Geometry check sheet. Reference: the model listing, model coordinates, mm. Face numbers are marked on the shaded views. A direction names the side the tool comes from. Round coordinates to 2 decimals unless told otherwise and drop trailing zeros. Loops run counter-clockwise (first coordinate to the right, second up) from the corner with the lowest first, then second, coordinate; pieces in that order, holes last.
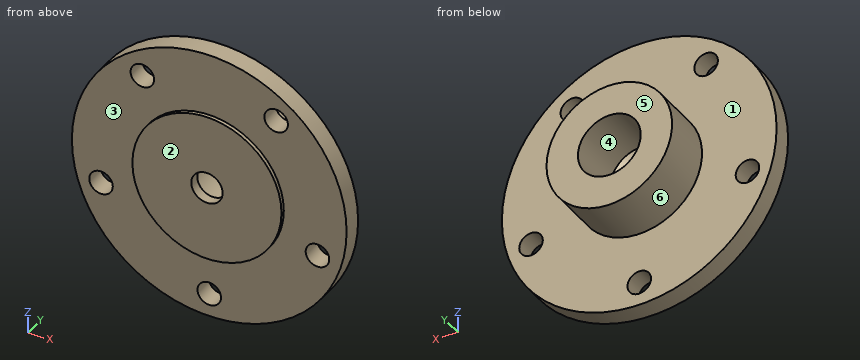
Autodesk Inventor part; units mm, degrees
ref_plane "YZ Plane" through (0, 0, 0) normal (1, 0, 0) x (0, 1, 0)
ref_plane "XZ Plane" through (0, 0, 0) normal (0, 1, 0) x (-1, 0, 0)
ref_plane "XY Plane" through (0, 0, 0) normal (0, 0, 1) x (1, 0, 0)
sketch "Sketch1" plane through (0, 0, 0) normal (0, 1, 0) x (-1, 0, 0)
  circle A0 centre (0, 0) radius 17.5
  dimension "d0" = 35
extrude "Extrusion1" add sketch "Sketch1" along normal mid plane 2.5
sketch "Sketch2" plane through (0, 1.25, 0) normal (0, 1, 0) x (1, 0, 0)
  circle A0 centre (0, 0) radius 8
  dimension "d3" = 16
extrude "Extrusion2" add sketch "Sketch2" along normal blind 6.5
sketch "Sketch3" plane through (0, -1.25, 0) normal (0, -1, 0) x (1, 0, 0)
  circle A0 centre (0, 0) radius 9.5
  dimension "d6" = 19
extrude "Extrusion3" add sketch "Sketch3" along normal blind 0.5
sketch "Sketch6" plane through (0, 1.25, 0) normal (0, 1, 0) x (1, 0, 0)
  circle A0 centre (0, 14.5) radius 1.5
  circle A1 centre (-13.7903, 4.4807) radius 1.5
  circle A2 centre (-8.5229, -11.7307) radius 1.5
  circle A3 centre (8.5229, -11.7307) radius 1.5
  circle A4 centre (13.7903, 4.4807) radius 1.5
  point P0 (0, 0)
  dimension "d17" = 3
  dimension "d18" = 14.5
  dimension "d21" = 360
extrude "Extrusion6" cut sketch "Sketch6" against normal through all
sketch "Sketch7" plane through (0, 7.75, 0) normal (0, 1, 0) x (1, 0, 0)
  point P0 (0, 0)
  point P1 (0, 0)
hole "Hole1" at (0, 7.75, 0) direction (0, -1, 0) diameter 8 depth 7 tip angle 118
sketch "Sketch8" plane through (0, -1.75, 0) normal (0, -1, 0) x (1, 0, 0)
  point P0 (0, 0)
hole "Hole2" at (0, -1.75, 0) direction (0, 1, 0) diameter 4 end through all
thread "Thread2"
properties material "Iron, Cast"
1) Access from +Z, -Z, +X, -X, +Y, -Y to the whole of each face (thin tool, end or side, straight path). Record for the marked faces 1, 2 and 3.
Report:
face 1: +Y
face 2: +Z, -Z, +X, -X, -Y
face 3: -Y
2) Mould release check, pull along X, two halves, no side actions. Record for the marked faces 4, 5 and 6: +X half, -X half, draft (parallel to the pull), parting line (faces both ways), or undercut.
Report:
face 4: undercut
face 5: draft
face 6: parting line
3) Scan lines: line 1 along Z through (x, y) = (0, 2.5); line 2 along Y through (x, z) = (9, 5); line 3 along Z through (x, y) = (1.5, 6.25). Record each from-to range of solid material in increasing order.
Report:
line 1: z = -8 to -4, 4 to 8
line 2: y = -1.25 to 1.25
line 3: z = -7.86 to -3.71, 3.71 to 7.86
4) Sectioned sample at A-A, the plane z = 0. Record the cut outline in (x, y).
Report:
outline: (-17.5, -1.25) - (-9.5, -1.25) - (-9.5, -1.75) - (-2, -1.75) - (-2, -0.45) - (-4, 0.75) - (-4, 7.75) - (-8, 7.75) - (-8, 1.25) - (-17.5, 1.25) - close; (2, -1.75) - (9.5, -1.75) - (9.5, -1.25) - (17.5, -1.25) - (17.5, 1.25) - (8, 1.25) - (8, 7.75) - (4, 7.75) - (4, 0.75) - (2, -0.45) - close
5) Sectioned sample at C-C, the plane x = -7.5. Record the cut outline in (y, z).
Report:
outline: (-1.75, -5.83) - (-1.25, -5.83) - (-1.25, -15.81) - (1.25, -15.81) - (1.25, -2.78) - (7.75, -2.78) - (7.75, 2.78) - (1.25, 2.78) - (1.25, 10.63) - (-1.25, 10.63) - (-1.25, 5.83) - (-1.75, 5.83) - close; (-1.25, 12.83) - (1.25, 12.83) - (1.25, 15.81) - (-1.25, 15.81) - close
6) Sectioned sample at B-B, the plane x = 0. Record the cut outline in (y, z), then the cut area to 3 significant figures.
Report:
outline: (-1.75, -9.5) - (-1.25, -9.5) - (-1.25, -13) - (1.25, -13) - (1.25, -8) - (7.75, -8) - (7.75, -4) - (0.75, -4) - (-0.45, -2) - (-1.75, -2) - close; (-1.75, 2) - (-0.45, 2) - (0.75, 4) - (7.75, 4) - (7.75, 8) - (1.25, 8) - (1.25, 17.5) - (-1.25, 17.5) - (-1.25, 9.5) - (-1.75, 9.5) - close; (-1.25, -17.5) - (1.25, -17.5) - (1.25, -16) - (-1.25, -16) - close
area: 125 mm2
7) Gauge pin test, flat ends, axial feed: pin 1 (5 mm diameter, centred on x = -8.52, z = 11.73, fed in from +Y); pin 2 (5 mm diameter, centred on x = -14, z = 4, fed in from -Y); pin 3 (1.5 mm diameter, centred on x = -13.5, y = 1.5, fed in from +Z); pin 4 (5 mm diameter, centred on x = 0, z = 0, fed in from -Y). Record the tip position at first contact, or that the pin passes through.
Report:
pin 1: stops at y = 1.25
pin 2: stops at y = -1.25
pin 3: stops at z = 11.94
pin 4: stops at y = -1.75
8) Sectioned sample at D-D, the plane y = 5.5. Record the cut outline in (x, z), then the cut area to 3 significant figures.
Report:
outline: circle Ø16 at (0, 0); hole circle Ø8 at (0, 0)
area: 151 mm2
